Autodesk Inventor part; units mm, degrees
ref_plane "YZ Plane" through (0, 0, 0) normal (1, 0, 0) x (0, 1, 0)
ref_plane "XZ Plane" through (0, 0, 0) normal (0, 1, 0) x (-1, 0, 0)
ref_plane "XY Plane" through (0, 0, 0) normal (0, 0, 1) x (1, 0, 0)
sketch "Sketch1" plane through (0, 0, 0) normal (1, 0, 0) x (0, 1, 0)
  line L0 (2, 0) -> (44, 0)
  line L1 (46, 2) -> (46, 30)
  line L2 (44, 32) -> (2, 32)
  line L3 (0, 30) -> (0, 2)
  arc A0 (2, 32) -> (0, 30) centre (2, 30) ccw
  arc A1 (46, 30) -> (44, 32) centre (44, 30) ccw
  arc A2 (44, 0) -> (46, 2) centre (44, 2) ccw
  arc A3 (0, 2) -> (2, 0) centre (2, 2) ccw
  line L4 (55.8524, 16) -> (-12.4215, 16) construction
  circle A4 centre (33.9212, 16) radius 4
  point P0 (0, 0)
  dimension "d3" = 8
extrude "Extrusion1" add sketch "Sketch1" along normal blind 23
extrude "Extrusion2" add sketch "Sketch1" along normal blind 41 contours A4
sketch "Sketch2" plane through (0, 0, 2) normal (0, -1, 0) x (1, 0, 0)
  line L0 (41, 10) -> (41, 18)
  line L1 (41, 14) -> (-14.7387, 14) construction
  circle A0 centre (10.7172, 12.4863) radius 12
  point P0 (0, -2)
  dimension "d12" = 24
extrude "Extrusion3" add sketch "Sketch2" along normal blind 31
properties part number "MOTOR 2"
For this review, take the finished solid that the model builds, in its own axes (mm). A direction names the side the tool comes from. Coordinates: 2 decimals unless noted, no trailing zeros. Order: outer loops, then holes, each group sorted by start corner. A loop starts at its lowest first (then second) coordinate and runs counter-clockwise, first axis right, second up. Notation, with made-up numbers: (21, 74) -> (38, 74) arc R22 cw to (38, 107) -> close; hole circle Ø2 at (52, 66). An arc over 180 degrees is marked (long way). Answer as CSV lines item,"result".
Q1. We need section D-D (z = 24.5). State the section outline as (x, y) points.
Model answer:
outline,"(0, 0) -> (4.1, 0) -> (4.1, -31) -> (17.33, -31) -> (17.33, 0) -> (23, 0) -> (23, 46) -> (0, 46) -> close"
Q2. For faces 4 (the face through (1.87, -15.28, 6.38)), 5 (the face through (31.874, 37.736, 14.799)), 6 (the face through (11.34, 0.6, 0.57)), list the 3-axis set-ups (+Z, -Z, +X, -X, +Y, -Y) from which the entire face can be reached by the end or side of a thin tool; tool diameter is ignored.
Model answer:
face 4,"-Y"
face 5,"+X"
face 6,"-Z, +X, -X, -Y"
Q3. We need section B-B (x = 25.5). State the section outline as (y, z) points, plus the area to 3 significant figures.
Model answer:
outline,"circle Ø8 at (33.92, 16)"
area,"50.3 mm2"
Q4. We need section A-A (z = 16). State the section outline as (x, y) points, plus the area to 3 significant figures.
Model answer:
outline,"(-1.19, -31) -> (22.62, -31) -> (22.62, 0) -> (23, 0) -> (23, 29.92) -> (41, 29.92) -> (41, 37.92) -> (23, 37.92) -> (23, 46) -> (0, 46) -> (0, 0) -> (-1.19, 0) -> close"
area,"1,940 mm2"
Q5. Clearance check with flat-ended pins moving along their axes: pin 1 Ø10 at (y, z) = (-7, 7.5) entering from -X; pin 2 Ø9.5 at (y, z) = (19.5, 20.5) entering from -X; pin 3 Ø1 at (x, z) = (-1, 16) entering from +Y. State where each tip first meets the part, or that it passes through.
Model answer:
pin 1,"stops at x = -1.12"
pin 2,"stops at x = 0"
pin 3,"stops at y = 0"
Q6. Draft analysis for pull direction X (two halves, no side actions). For faces 1 (the face through (11, 46, 16)), 2 (the face through (0, 23, 16)), 3 (the face through (41, 34, 16)), state which applies: released by +X, released by -X, zero draft, split by the parting line, or undercut.
Model answer:
face 1,"zero draft"
face 2,"released by -X"
face 3,"released by +X"
Q7. Wall thickness on line 1 along X through (y, z) = (28, 29); line 2 along Y through (x, z) = (5, 27); line 3 along Z through (x, y) = (37.5, 36.5): over which ranges is each line inside the solid? List them lowest first. Write a range as [from, to].
Model answer:
line 1,"x = [0, 23]"
line 2,"y = [0, 46]"
line 3,"z = [12.94, 19.06]"
Q8. We need section C-C (y = 24). State the section outline as (x, z) points.
Model answer:
outline,"(0, 0) -> (23, 0) -> (23, 32) -> (0, 32) -> close"
